Autodesk Inventor part; units mm, degrees
ref_plane "YZ Plane" through (0, 0, 0) normal (1, 0, 0) x (0, 1, 0)
ref_plane "XZ Plane" through (0, 0, 0) normal (0, 1, 0) x (-1, 0, 0)
ref_plane "XY Plane" through (0, 0, 0) normal (0, 0, 1) x (1, 0, 0)
sketch "Sketch1" plane through (0, 0, 0) normal (0, 0, 1) x (1, 0, 0)
  line L0 (53.5, -12.0505) -> (-53.5, -12.0505)
  line L1 (-57.5, -8.0505) -> (-57.5, 78.4495)
  line L2 (-53.5, 82.4495) -> (53.5, 82.4495)
  line L3 (57.5, 78.4495) -> (57.5, -8.0505)
  line L4 (57.5, -12.0505) -> (-57.5, 82.4495) construction
  line L5 (-57.5, -12.0505) -> (57.5, 82.4495) construction
  arc A0 (-53.5, 82.4495) -> (-57.5, 78.4495) centre (-53.5, 78.4495) ccw
  arc A1 (57.5, 78.4495) -> (53.5, 82.4495) centre (53.5, 78.4495) ccw
  arc A2 (53.5, -12.0505) -> (57.5, -8.0505) centre (53.5, -8.0505) ccw
  arc A3 (-57.5, -8.0505) -> (-53.5, -12.0505) centre (-53.5, -8.0505) ccw
  point P0 (0, 0)
  point P1 (0, 35.1995)
  dimension "d0" = 115
  dimension "d1" = 94.5
  dimension "d2" = 4
extrude "Extrusion1" add sketch "Sketch1" along normal blind 15
sketch "Sketch2" plane through (0, 0, 15) normal (0, 0, 1) x (1, 0, 0)
  line L0 (53.5, 82.4495) -> (-53.5, 82.4495)
  arc A0 (-53.5, 82.4495) -> (-57.5, 78.4495) centre (-53.5, 78.4495) ccw
  line L1 (-57.5, 78.4495) -> (-57.5, -8.0505)
  arc A1 (-57.5, -8.0505) -> (-53.5, -12.0505) centre (-53.5, -8.0505) ccw
  line L2 (-53.5, -12.0505) -> (53.5, -12.0505)
  arc A2 (53.5, -12.0505) -> (57.5, -8.0505) centre (53.5, -8.0505) ccw
  line L3 (57.5, -8.0505) -> (57.5, 78.4495)
  arc A3 (57.5, 78.4495) -> (53.5, 82.4495) centre (53.5, 78.4495) ccw
  line L4 (-53.5, 93.4495) -> (53.5, 93.4495)
  arc A4 (68.5, 78.4495) -> (53.5, 93.4495) centre (53.5, 78.4495) ccw
  line L5 (68.5, 78.4495) -> (68.5, -8.0505)
  arc A5 (53.5, -23.0505) -> (68.5, -8.0505) centre (53.5, -8.0505) ccw
  line L6 (53.5, -23.0505) -> (-53.5, -23.0505)
  arc A6 (-68.5, -8.0505) -> (-53.5, -23.0505) centre (-53.5, -8.0505) ccw
  line L7 (-68.5, -8.0505) -> (-68.5, 78.4495)
  arc A7 (-53.5, 93.4495) -> (-68.5, 78.4495) centre (-53.5, 78.4495) ccw
  circle A8 centre (-32.5, 91.4495) radius 1.5
  circle A9 centre (33.5, 91.4495) radius 1.5
  circle A10 centre (64.5, 64.6495) radius 1.5
  circle A11 centre (64.5, 4.6495) radius 1.5
  point P0 (0, 0)
  dimension "d5" = 11
  dimension "d6" = 3
  dimension "d7" = 3
  dimension "d8" = 3
  dimension "d9" = 3
  dimension "d10" = 24
  dimension "d11" = 66
  dimension "d12" = 9
  dimension "d13" = 7
  dimension "d14" = 7
  dimension "d15" = 17.8
  dimension "d16" = 60
extrude "Extrusion2" add sketch "Sketch2" along normal blind 2 contours A3 L3 A2 L2 A1 L1 A0 L0 | L4 A4 L5 A5 L6 A6 L7 A7
sketch "Sketch3" plane through (0, 0, 15) normal (0, 0, -1) x (-1, 0, 0)
  circle A0 centre (-64.5, 4.6495) radius 1.5
  circle A1 centre (-64.5, 64.6495) radius 1.5
  circle A2 centre (-33.5, 91.4495) radius 1.5
  circle A3 centre (32.5, 91.4495) radius 1.5
  line L0 (53.5, -23.0505) -> (-53.5, -23.0505)
  arc A4 (53.5, -23.0505) -> (68.5, -8.0505) centre (53.5, -8.0505) ccw
  line L1 (68.5, 78.4495) -> (68.5, -8.0505)
  arc A5 (68.5, 78.4495) -> (53.5, 93.4495) centre (53.5, 78.4495) ccw
  line L2 (-53.5, 93.4495) -> (53.5, 93.4495)
  arc A6 (-53.5, 93.4495) -> (-68.5, 78.4495) centre (-53.5, 78.4495) ccw
  line L3 (-68.5, -8.0505) -> (-68.5, 78.4495)
  arc A7 (-68.5, -8.0505) -> (-53.5, -23.0505) centre (-53.5, -8.0505) ccw
  arc A8 (-53.5, 82.4495) -> (-57.5, 78.4495) centre (-53.5, 78.4495) ccw
  line L4 (-53.5, 82.4495) -> (53.5, 82.4495)
  arc A9 (57.5, 78.4495) -> (53.5, 82.4495) centre (53.5, 78.4495) ccw
  line L5 (57.5, 78.4495) -> (57.5, -8.0505)
  arc A10 (53.5, -12.0505) -> (57.5, -8.0505) centre (53.5, -8.0505) ccw
  line L6 (53.5, -12.0505) -> (-53.5, -12.0505)
  arc A11 (-57.5, -8.0505) -> (-53.5, -12.0505) centre (-53.5, -8.0505) ccw
  line L7 (-57.5, -8.0505) -> (-57.5, 78.4495)
  arc A12 (-53.5, 93.4495) -> (-68.5, 78.4495) centre (-53.5, 78.4495) ccw
  line L8 (-57.5, -8.0505) -> (-57.5, 78.4495)
  line L9 (-68.5, 78.4495) -> (-57.5, 78.4495)
  line L10 (-57.5, 78.4495) -> (-57.5, -8.0505)
  line L11 (-57.5, -8.0505) -> (-68.5, -8.0505)
  line L12 (-68.5, -8.0505) -> (-68.5, 78.4495)
  point P0 (0, 0)
  point P1 (-68.5, -0.3835)
extrude "Extrusion3" add sketch "Sketch3" along normal blind 2.5 contours L3 L9 L7 L11
sketch "Sketch4" plane through (0, 0, 17) normal (0, 0, 1) x (1, 0, 0)
  line L0 (53.5, 82.4495) -> (-53.5, 82.4495)
  arc A0 (57.5, 78.4495) -> (53.5, 82.4495) centre (53.5, 78.4495) ccw
  line L1 (57.5, -8.0505) -> (57.5, 78.4495)
  arc A1 (53.5, -12.0505) -> (57.5, -8.0505) centre (53.5, -8.0505) ccw
  line L2 (-53.5, -12.0505) -> (53.5, -12.0505)
  arc A2 (-57.5, -8.0505) -> (-53.5, -12.0505) centre (-53.5, -8.0505) ccw
  line L3 (-57.5, 78.4495) -> (-57.5, -8.0505)
  arc A3 (-53.5, 82.4495) -> (-57.5, 78.4495) centre (-53.5, 78.4495) ccw
  line L4 (-53.5, 79.4495) -> (53.5, 79.4495)
  arc A4 (54.5, 78.4495) -> (53.5, 79.4495) centre (53.5, 78.4495) ccw
  line L5 (54.5, 78.4495) -> (54.5, -8.0505)
  arc A5 (53.5, -9.0505) -> (54.5, -8.0505) centre (53.5, -8.0505) ccw
  line L6 (53.5, -9.0505) -> (-53.5, -9.0505)
  arc A6 (-54.5, -8.0505) -> (-53.5, -9.0505) centre (-53.5, -8.0505) ccw
  line L7 (-54.5, -8.0505) -> (-54.5, 78.4495)
  arc A7 (-53.5, 79.4495) -> (-54.5, 78.4495) centre (-53.5, 78.4495) ccw
  point P0 (0, 0)
  dimension "d21" = 3
extrude "Extrusion4" cut sketch "Sketch4" against normal blind 14 contours L4 A4 L5 A5 L6 A6 L7 A7
sketch "Sketch7" plane through (0, 0, 17) normal (0, 0, 1) x (1, 0, 0)
  arc A0 (53.5, -9.0505) -> (54.5, -8.0505) centre (53.5, -8.0505) ccw
  line L0 (53.5, -9.0505) -> (-53.5, -9.0505)
  arc A1 (-54.5, -8.0505) -> (-53.5, -9.0505) centre (-53.5, -8.0505) ccw
  line L1 (-54.5, -8.0505) -> (-54.5, 78.4495)
  arc A2 (-53.5, 79.4495) -> (-54.5, 78.4495) centre (-53.5, 78.4495) ccw
  line L2 (-53.5, 79.4495) -> (53.5, 79.4495)
  arc A3 (54.5, 78.4495) -> (53.5, 79.4495) centre (53.5, 78.4495) ccw
  line L3 (54.5, 78.4495) -> (54.5, -8.0505)
  line L4 (-53.5, -23.0505) -> (53.5, -23.0505)
  arc A4 (53.5, -23.0505) -> (68.5, -8.0505) centre (53.5, -8.0505) ccw
  line L5 (68.5, -8.0505) -> (68.5, 78.4495)
  arc A5 (68.5, 78.4495) -> (53.5, 93.4495) centre (53.5, 78.4495) ccw
  line L6 (53.5, 93.4495) -> (-53.5, 93.4495)
  arc A6 (-53.5, 93.4495) -> (-68.5, 78.4495) centre (-53.5, 78.4495) ccw
  line L7 (-68.5, 78.4495) -> (-68.5, -8.0505)
  arc A7 (-68.5, -8.0505) -> (-53.5, -23.0505) centre (-53.5, -8.0505) ccw
  circle A8 centre (-32.5, 91.4495) radius 1.5
  circle A9 centre (33.5, 91.4495) radius 1.5
  circle A10 centre (64.5, 64.6495) radius 1.5
  circle A11 centre (64.5, 4.6495) radius 1.5
  line L8 (-53.5, -12.0505) -> (53.5, -12.0505)
  line L9 (-75.3145, -26.4449) -> (0.399, -26.4449)
  line L10 (0.399, -26.4449) -> (0.399, -12.0505)
  line L11 (0.399, -12.0505) -> (-75.3145, -12.0505)
  line L12 (-75.3145, -12.0505) -> (-75.3145, -26.4449)
  point P0 (0, 0)
extrude "Extrusion7" cut sketch "Sketch7" against normal through all contours A7 L11 L8 L10 L4 | L4 L10 L9 L12 L11 A7
fillet "Fillet1" radius 2 10 edges at (56.3284, -10.8789, 0) (57.5, 35.1995, 0) (56.3284, 81.2779, 0) (0, 82.4495, 0) (-56.3284, 81.2779, 0) (-57.5, 35.1995, 0) (-56.3284, -10.8789, 0) (0, -12.0505, 0) (0.399, -12.0505, 16) (0.399, -23.0505, 16)
sketch "Sketch8" plane through (0, 0, 17) normal (0, 0, 1) x (1, 0, 0)
  circle A0 centre (64.5, 64.6495) radius 1.5
  circle A1 centre (64.5, 4.6495) radius 1.5
  circle A2 centre (-95.5, 64.6495) radius 1.5
  circle A3 centre (-95.5, 4.6495) radius 1.5
  arc A4 (0.399, -21.0505) -> (2.399, -23.0505) centre (2.399, -21.0505) ccw
  line L0 (2.399, -23.0505) -> (53.5, -23.0505)
  arc A5 (53.5, -23.0505) -> (68.5, -8.0505) centre (53.5, -8.0505) ccw
  line L1 (68.5, -8.0505) -> (68.5, 78.4495)
  arc A6 (68.5, 78.4495) -> (53.5, 93.4495) centre (53.5, 78.4495) ccw
  line L2 (53.5, 93.4495) -> (-53.5, 93.4495)
  arc A7 (-53.5, 93.4495) -> (-68.5, 78.4495) centre (-53.5, 78.4495) ccw
  line L3 (-68.5, 78.4495) -> (-68.5, -8.0505)
  arc A8 (-68.5, -8.0505) -> (-68.3214, -10.3582) centre (-53.5, -8.0505) ccw
  arc A9 (-68.3214, -10.3582) -> (-66.3452, -12.0505) centre (-66.3452, -10.0505) ccw
  line L4 (-66.3452, -12.0505) -> (-1.601, -12.0505)
  arc A10 (0.399, -14.0505) -> (-1.601, -12.0505) centre (-1.601, -14.0505) ccw
  line L5 (0.399, -14.0505) -> (0.399, -21.0505)
  arc A11 (53.5, -9.0505) -> (54.5, -8.0505) centre (53.5, -8.0505) ccw
  line L6 (53.5, -9.0505) -> (-53.5, -9.0505)
  arc A12 (-54.5, -8.0505) -> (-53.5, -9.0505) centre (-53.5, -8.0505) ccw
  line L7 (-54.5, -8.0505) -> (-54.5, 78.4495)
  arc A13 (-53.5, 79.4495) -> (-54.5, 78.4495) centre (-53.5, 78.4495) ccw
  line L8 (-53.5, 79.4495) -> (53.5, 79.4495)
  arc A14 (54.5, 78.4495) -> (53.5, 79.4495) centre (53.5, 78.4495) ccw
  line L9 (54.5, 78.4495) -> (54.5, -8.0505)
  circle A15 centre (-32.5, 91.4495) radius 1.5
  circle A16 centre (33.5, 91.4495) radius 1.5
  circle A17 centre (64.5, 64.6495) radius 1.5
  circle A18 centre (64.5, 4.6495) radius 1.5
  line L10 (-106.5344, -10.0505) -> (-106.5344, 73.4495)
  arc A19 (-86.5344, 93.4495) -> (-106.5344, 73.4495) centre (-86.5344, 73.4495) ccw
  line L11 (-53.5, 93.4495) -> (-86.5344, 93.4495)
  line L12 (-53.5, -12.0505) -> (-66.3452, -12.0505)
  line L13 (-66.3452, -12.0505) -> (-104.5344, -12.0505)
  arc A20 (-106.5344, -10.0505) -> (-104.5344, -12.0505) centre (-104.5344, -10.0505) ccw
  point P0 (0, 0)
  dimension "d37" = 3
  dimension "d38" = 3
  dimension "d39" = 160
  dimension "d40" = 0
  dimension "d41" = 0
  dimension "d42" = 2
  dimension "d54" = 20
extrude "Extrusion8" add sketch "Sketch8" against normal up to surface (2 mm away) contours L13 A20 L10 A19 L11 A7 L3 A8 A9
sketch "Skizze9" plane through (0, 0, 3) normal (0, 0, 1) x (1, 0, 0)
  line L0 (53.5, -9.0505) -> (-53.5, -9.0505)
  arc A0 (53.5, -9.0505) -> (54.5, -8.0505) centre (53.5, -8.0505) ccw
  line L1 (54.5, 78.4495) -> (54.5, -8.0505)
  arc A1 (54.5, 78.4495) -> (53.5, 79.4495) centre (53.5, 78.4495) ccw
  line L2 (-53.5, 79.4495) -> (53.5, 79.4495)
  arc A2 (-53.5, 79.4495) -> (-54.5, 78.4495) centre (-53.5, 78.4495) ccw
  line L3 (-54.5, -8.0505) -> (-54.5, 78.4495)
  arc A3 (-54.5, -8.0505) -> (-53.5, -9.0505) centre (-53.5, -8.0505) ccw
  circle A4 centre (0, 35.1995) radius 15
  point P0 (0, 0)
  dimension "d45" = 30
extrude "Extrusion9" cut sketch "Skizze9" against normal blind 13 contours A4
sketch "Skizze10" plane through (0, 0, 3) normal (0, 0, 1) x (1, 0, 0)
  circle A0 centre (19.4922, 35.1995) radius 4
  circle A1 centre (-9.7461, 52.0802) radius 4
  circle A2 centre (-9.7461, 18.3188) radius 4
  circle A3 centre (9.7461, 52.0802) radius 1.45
  circle A4 centre (9.7461, 18.3188) radius 1.45
  circle A5 centre (-19.4922, 35.1995) radius 1.45
  circle A6 centre (0, 35.1995) radius 13.5
  circle A7 centre (0, 35.1995) radius 23.9428
  circle A8 centre (19.4922, 35.1995) radius 1.4
  point P0 (0, 0)
  dimension "d48" = 2.8
extrude "Extrusion10" cut sketch "Skizze10" against normal blind 14 contours A8
pattern_circular "Runde Anordnung1" count 6 over 360 about axis through (0, 35.1995, 3) along (0, 0, -1) of "Extrusion10"
properties part number "30_XYTable_Aliexpress_sampleinsert_round"
Geometry check sheet. Reference: the model listing, model coordinates, mm. A direction names the side the tool comes from. Give positions to 0.01 mm unless a question says otherwise; leave off trailing zeros. Order: outer loops, then holes, each group sorted by start corner. A loop starts at its lowest first (then second) coordinate and runs counter-clockwise, first axis right, second up. Notation, with made-up numbers: M 40,-25 L 53,-25 A16 cw 53,-6 Z; hole C 82.5,-19 d9. An arc over 180 degrees is marked long. Use a Markdown table: item, result.
Item 1: Depth check by flat-ended pin: P1, Ø6, axis at y = 54.5, z = 11.5, coming from the -X side; P2, Ø2.5, axis at x = -95.5, y = 64.65, coming from the -Z side; P3, Ø4, axis at y = 79, z = 7.5, coming from the +X side; P4, Ø3, axis at x = 61, z = 14, coming from the +Y side. Enter the tip coordinate at first touch or a pass-through.
Answers follow:
| item | result |
|---|---|
| P1 | stops at x = -57.5 |
| P2 | passes through |
| P3 | stops at x = 57.5 |
| P4 | stops at y = 92.02 |
Item 2: Section check A-A (z = 7). Record the cut outline in (x, y), and give its area (3 significant figures).
Answers follow:
| item | result |
|---|---|
| outline | M -57.5,-8.05 A4 ccw -53.5,-12.05 L 53.5,-12.05 A4 ccw 57.5,-8.05 L 57.5,78.45 A4 ccw 53.5,82.45 L -53.5,82.45 A4 ccw -57.5,78.45 Z; hole M -54.5,-8.05 A1 ccw -53.5,-9.05 L 53.5,-9.05 A1 ccw 54.5,-8.05 L 54.5,78.45 A1 ccw 53.5,79.45 L -53.5,79.45 A1 ccw -54.5,78.45 Z |
| area | 1,210 mm2 |
Item 3: Section check B-B (y = 38.5). Record the cut outline in (x, z), and give its area (3 significant figures).
Answers follow:
| item | result |
|---|---|
| outline | M -106.53,15 L -57.5,15 L -57.5,2 A2 ccw -55.5,0 L -14.63,0 L -14.63,3 L -54.5,3 L -54.5,17 L -106.53,17 Z; M 14.63,0 L 55.5,0 A2 ccw 57.5,2 L 57.5,12.5 L 68.5,12.5 L 68.5,17 L 54.5,17 L 54.5,3 L 14.63,3 Z |
| area | 487 mm2 |
Item 4: Material ranges on line 1 along X through (y, z) = (46.5, 7); line 2 along Y through (x, z) = (39, 7.5); line 3 along X through (y, z) = (44, 14), recorded low to high.
Answers follow:
| item | result |
|---|---|
| line 1 | x = -57.5 to -54.5, 54.5 to 57.5 |
| line 2 | y = -12.05 to -9.05, 79.45 to 82.45 |
| line 3 | x = -57.5 to -54.5, 54.5 to 68.5 |
Item 5: Section check D-D (x = 43.5). Record the cut outline in (y, z).
Answers follow:
| item | result |
|---|---|
| outline | M -23.05,15 L -12.05,15 L -12.05,2 A2 ccw -10.05,0 L 80.45,0 A2 ccw 82.45,2 L 82.45,15 L 93.45,15 L 93.45,17 L 79.45,17 L 79.45,3 L -9.05,3 L -9.05,17 L -23.05,17 Z |
Item 6: Section check C-C (y = 69). Record the cut outline in (x, z), and give its area (3 significant figures).
Answers follow:
| item | result |
|---|---|
| outline | M -106.53,15 L -57.5,15 L -57.5,2 A2 ccw -55.5,0 L 55.5,0 A2 ccw 57.5,2 L 57.5,12.5 L 68.5,12.5 L 68.5,17 L 54.5,17 L 54.5,3 L -54.5,3 L -54.5,17 L -106.53,17 Z |
| area | 575 mm2 |
Item 7: Tool access check on faces 4 (the flat face through (-1, 82.45, 8)), 5 (the cylindrical face through (-56.359, 81.247, 8.409)), 6 (the flat face through (54.5, 36, 10)), 7 (the flat face through (-57.5, 35, 8)), 8 (the flat face through (57.5, 36, 7)). Record the directions out of +Z, -Z, +X, -X, +Y, -Y that give a thin tool (end or side, any length) a straight path to the whole face; none if there is none.
Answers follow:
| item | result |
|---|---|
| face 4 | -Z, +X, -X, +Y |
| face 5 | -Z, -X, +Y |
| face 6 | +Z |
| face 7 | -Z, -X, +Y, -Y |
| face 8 | -Z, +X, +Y, -Y |
Item 8: Draft check along Y on faces 1 (the flat face through (-13, 46, 0)), 2 (the cylindrical face through (63.99, 89.17, 15.99)), 3 (the flat face through (-13, 46, 3)). Enter one of: +Y half, -Y half, draft (parallel to the pull), parting line (faces both ways), or undercut.
Answers follow:
| item | result |
|---|---|
| face 1 | draft |
| face 2 | +Y half |
| face 3 | undercut |
